Model file for the job. Use its own axes, mm. A direction names the side the tool comes from. Give positions to 0.01 mm unless a question says otherwise; leave off trailing zeros. Write each loop counter-clockwise with the first axis right and the second up, starting at its lowest first coordinate (ties: lowest second). Pieces come first, ordered by that corner, then holes.
```python
from build123d import *

# Parameters (mm, degrees)
F0_W     = 30.988
F0_H     = 6.35
F1_DEPTH = 1.524
F2_R     = 1.9304
F3_DEPTH = 0.762
F4_R     = 1.27
F5_DEPTH = 0.762
F6_W     = 7.62
F6_H     = 6.35
F7_DEPTH = 5.08
F8_R     = 1.651
F9_DEPTH = 5.08


with BuildPart() as f1:
    # F0 (on Top) → F1 (new body)
    with BuildSketch(Plane.XY):
        Rectangle(F0_W, F0_H)
    extrude(amount=F1_DEPTH)

    # F2 (on face) → F3 (cut)
    with BuildSketch(Plane.XY.offset(1.524)):
        with Locations((-8.6868, 0)):
            Circle(F2_R)
        with Locations((8.6868, 0)):
            Circle(F2_R)
    extrude(amount=-F3_DEPTH, mode=Mode.SUBTRACT)

    # F4 (on face) → F5 (cut)
    with BuildSketch(Plane.XY.offset(0.762)):
        with Locations((-8.6868, 0)):
            Circle(F4_R)
        with Locations((8.6868, 0)):
            Circle(F4_R)
    extrude(amount=-F5_DEPTH, mode=Mode.SUBTRACT)

    # F6 (on face) → F7 (join)
    with BuildSketch(Plane.XY.offset(1.524)):
        Rectangle(F6_W, F6_H)
    extrude(amount=F7_DEPTH)

    # F8 (on face) → F9 (cut)
    with BuildSketch(Plane.XY.offset(6.604)):
        Circle(F8_R)
    extrude(amount=-F9_DEPTH, mode=Mode.SUBTRACT)


solid = f1.part
```
1. Which spindle directions (+Z, -Z, +X, -X, +Y, -Y) get a long thin tool onto all of the face, cutting with end or side? Do faces 4 (the flat face through (-11, 0, 1.524)), 5 (the cylindrical face through (7.42, 0.06, 0.39)), 6 (the flat face through (3.81, 0, 4)), 7 (the cylindrical face through (-6.846, 0.58, 1.148)). Say none if no direction does.
Calculated:
face 4: +Z, -X, +Y, -Y
face 5: +Z, -Z
face 6: +Z, +X, +Y, -Y
face 7: +Z
2. Slice it at A-A, the plane y = 0. Write the cut outline in (x, z), and give its area (3 significant figures).
Calculated:
outline: (-15.49, 0) - (-9.96, 0) - (-9.96, 0.76) - (-10.62, 0.76) - (-10.62, 1.52) - (-15.49, 1.52) - close; (-7.42, 0) - (7.42, 0) - (7.42, 0.76) - (6.76, 0.76) - (6.76, 1.52) - (3.81, 1.52) - (3.81, 6.6) - (1.65, 6.6) - (1.65, 1.52) - (-1.65, 1.52) - (-1.65, 6.6) - (-3.81, 6.6) - (-3.81, 1.52) - (-6.76, 1.52) - (-6.76, 0.76) - (-7.42, 0.76) - close; (9.96, 0) - (15.49, 0) - (15.49, 1.52) - (10.62, 1.52) - (10.62, 0.76) - (9.96, 0.76) - close
area: 59.4 mm2
3. Probe probe 1 along Y at (x, z) = (0, 5) (3 decimals); probe 2 along X at (y, z) = (-1.75, 5.25); probe 3 along Z at (x, y) = (-6, -2). List the from-to ranges inside material, lowest first.
Calculated:
probe 1: y = -3.175 to -1.651, 1.651 to 3.175
probe 2: x = -3.81 to 3.81
probe 3: z = 0 to 1.52
4. Slice it at B-B, the plane x = 0. Write the cut outline in (y, z) (3 decimals).
Calculated:
outline: (-3.175, 0) - (3.175, 0) - (3.175, 6.604) - (1.651, 6.604) - (1.651, 1.524) - (-1.651, 1.524) - (-1.651, 6.604) - (-3.175, 6.604) - close
5. Slice it at C-C, the plane z = 4. Write the cut outline in (x, y) (3 decimals), and give its area (3 significant figures).
Calculated:
outline: (-3.81, -3.175) - (3.81, -3.175) - (3.81, 3.175) - (-3.81, 3.175) - close; hole circle Ø3.302 at (0, 0)
area: 39.8 mm2
6. Slice it at D-D, the plane y = 2.75. Write the cut outline in (x, z).
Calculated:
outline: (-15.49, 0) - (15.49, 0) - (15.49, 1.52) - (3.81, 1.52) - (3.81, 6.6) - (-3.81, 6.6) - (-3.81, 1.52) - (-15.49, 1.52) - close
7. Pin check, flat tips, straight feed: P1, Ø1.9, axis at x = 9, y = 0.5, coming from the +Z side; P2, Ø1.5, axis at y = -1, z = 4.5, coming from the +X side; P3, Ø1.7, axis at x = 0, y = 0.5, coming from the +Z side. Stop position of each tip, or through.
Calculated:
P1: stops at z = 0.76
P2: stops at x = 3.81
P3: stops at z = 1.52
8. Pull direction Y, two halves, no side cores. Call faces 1 (the flat face through (15.494, 0, 1)), 2 (the flat face through (0, -3.175, 3)), 3 (the cylindrical face through (-9.956, 0.056, 0.386)): +Y half, -Y half, draft (parallel to the pull), parting line (faces both ways), or undercut.
Calculated:
face 1: draft
face 2: -Y half
face 3: undercut
